```python
from build123d import *

# Parameters (mm, degrees)
CROQUIS1_R              = 3.75
CROQUIS1_R_2            = 2.5
SALIENTE_EXTRUIR1_DEPTH = 22.5


with BuildPart() as part:
    # Croquis1 → Saliente-Extruir1 (new body)
    with BuildSketch(Plane.XY):
        with Locations((1, 53.5)):
            Circle(CROQUIS1_R)
        with Locations((1, 53.5)):
            Circle(CROQUIS1_R_2, mode=Mode.SUBTRACT)
        with BuildLine():
            Line((0, 49.885791926), (0, 0))
            Line((0, 0), (2, 7.5))
            Line((2, 7.5), (2, 49.885791926))
            ThreePointArc((2, 49.885791926), (1, 49.75), (0, 49.885791926))
        make_face()
    extrude(amount=SALIENTE_EXTRUIR1_DEPTH)


solid = part.part
```
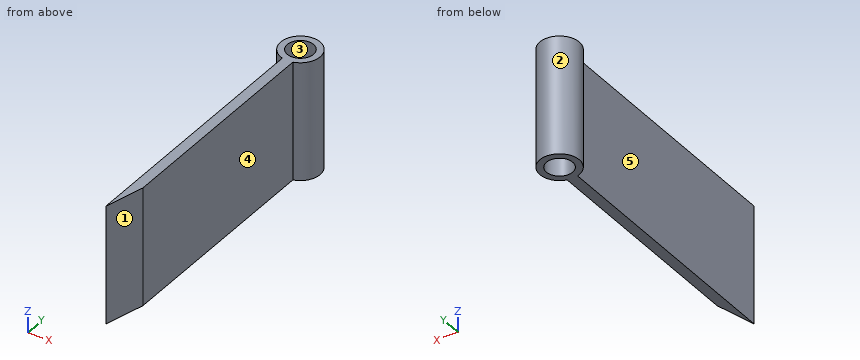
CAD build for the part. Positions are in the model's coordinates, mm. Face numbers are marked on the shaded views. A direction names the side the tool comes from. Round coordinates to 2 decimals unless told otherwise and drop trailing zeros. Order: outer loops, then holes, each group sorted by start corner. A loop starts at its lowest first (then second) coordinate and runs counter-clockwise, first axis right, second up.
Item 1: Saw through at D-D on y = 21. Write the cut outline in (x, z).
Item 2: Saw through at A-A on x = 1. Write the cut outline in (y, z), then the cut area to 3 significant figures.
Item 3: Saw through at B-B on y = 53.5. Write the cut outline in (x, z).
Item 4: Mould opens along X. For the marked faces 1, 2 and 3 say: pulls with the +X half, pulls with the -X half, needs draft (parallel to the pull), parting line crosses it, or undercut.
Item 5: Tool access for the marked faces 4 and 5: list every direction of +Z, -Z, +X, -X, +Y, -Y with a clear straight run to the whole face (end or side of a thin tool).
Item 6: Pin check, flat tips, straight feed: pin 1 (1 mm diameter, centred on x = -1.5, z = 20, fed in from +Y); pin 2 (4.5 mm diameter, centred on x = 1, y = 53.5, fed in from +Z); pin 3 (7 mm diameter, centred on y = 18.5, z = 14.5, fed in from +X). Stop position of each tip, or through.
Item 7: Saw through at C-C on z = 18.25. Write the cut outline in (x, y).
Item 8: Probe line 1 along X through (y, z) = (45, 16.5); line 2 along Y through (x, z) = (-0.5, 3.5); line 3 along Y through (x, z) = (-0.75, 3.5). List the from-to ranges inside material, lowest first.
Reported:
1. outline: (0, 0) - (2, 0) - (2, 22.5) - (0, 22.5) - close
2. outline: (3.75, 0) - (51, 0) - (51, 22.5) - (3.75, 22.5) - close; (56, 0) - (57.25, 0) - (57.25, 22.5) - (56, 22.5) - close
2. area: 1,090 mm2
3. outline: (-2.75, 0) - (-1.5, 0) - (-1.5, 22.5) - (-2.75, 22.5) - close; (3.5, 0) - (4.75, 0) - (4.75, 22.5) - (3.5, 22.5) - close
4. face 1: pulls with the +X half
4. face 2: parting line crosses it
4. face 3: undercut
5. face 4: +Z, -Z, +X, -Y
5. face 5: +Z, -Z, -X, -Y
6. pin 1: stops at y = 56.67
6. pin 2: passes through
6. pin 3: stops at x = 2
7. outline: (0, 0) - (2, 7.5) - (2, 49.89) arc R3.75 ccw (long way) to (0, 49.89) - close; hole circle Ø5 at (1, 53.5)
8. line 1: x = 0 to 2
8. line 2: y = 50.06 to 51.5, 55.5 to 56.94
8. line 3: y = 50.18 to 51.71, 55.29 to 56.82
